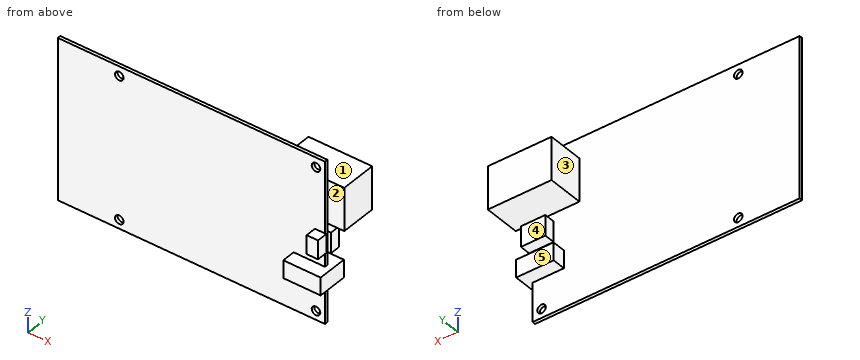
from build123d import *

# Parameters (mm, degrees)
ESQUISSE1_W             = 100
ESQUISSE1_H             = 60
BOSS_EXTRU_1_DEPTH      = 1.2
ESQUISSE2_W             = 21.84
ESQUISSE2_H             = 16
BOSS_EXTRU_2_DEPTH      = 13.5
ESQUISSE3_W             = 9.16
ESQUISSE3_H             = 7.62
BOSS_EXTRU_3_DEPTH      = 4
BOSS_EXTRU_4_DEPTH      = 5
BOSS_EXTRU_4_DEPTH_BACK = 6.2
ESQUISSE4_W             = 14
ESQUISSE4_H             = 6.6
ESQUISSE5_W             = 4.25
ESQUISSE5_H             = 7
BOSS_EXTRU_5_DEPTH      = 4
ENL_V_MAT_EXTRU_1_REACH = 119.398
ESQUISSE6_R             = 1.6
ESQUISSE7_W             = 16
ESQUISSE7_H             = 13.5
BOSS_EXTRU_6_DEPTH      = 2


with BuildPart() as part:
    # Esquisse1 → Boss.-Extru.1 (new body)
    with BuildSketch(Plane(origin=(0, 0, 0), x_dir=(1, 0, 0), z_dir=(0, 1, 0))):
        with Locations((-50, 30)):
            Rectangle(ESQUISSE1_W, ESQUISSE1_H)
    extrude(amount=-BOSS_EXTRU_1_DEPTH)

    # Esquisse2 → Boss.-Extru.2 (add)
    with BuildSketch(Plane(origin=(0, 0, 0), x_dir=(1, 0, 0), z_dir=(0, 1, 0))):
        with Locations((-6.62, 15.5)):
            Rectangle(ESQUISSE2_W, ESQUISSE2_H)
    extrude(amount=BOSS_EXTRU_2_DEPTH)

    # Esquisse3 → Boss.-Extru.3 (add)
    with BuildSketch(Plane(origin=(0, 0, 0), x_dir=(1, 0, 0), z_dir=(0, 1, 0))):
        with Locations((-3.29, 30.18)):
            Rectangle(ESQUISSE3_W, ESQUISSE3_H)
    extrude(amount=BOSS_EXTRU_3_DEPTH)

    # Esquisse4 → Boss.-Extru.4 (add, two sides: drawn at the far end of the back side and taken through both)
    with BuildSketch(Plane(origin=(0, 0, 0), x_dir=(1, 0, 0), z_dir=(0, 1, 0)).offset(-BOSS_EXTRU_4_DEPTH_BACK)):
        with Locations((-4.736, 42.16)):
            Rectangle(ESQUISSE4_W, ESQUISSE4_H)
    extrude(amount=BOSS_EXTRU_4_DEPTH + BOSS_EXTRU_4_DEPTH_BACK)

    # Esquisse5 → Boss.-Extru.5 (add)
    with BuildSketch(Plane.XZ.offset(1.2)):
        with Locations((-1.625, -30.01)):
            Rectangle(ESQUISSE5_W, ESQUISSE5_H)
    extrude(amount=BOSS_EXTRU_5_DEPTH)

    # Esquisse6 → Enlèv. mat.-Extru.1 (cut, up to next)
    with BuildSketch(Plane(origin=(0, 0, 0), x_dir=(1, 0, 0), z_dir=(0, 1, 0)), mode=Mode.PRIVATE) as enl_v_mat_extru_1_sk1:
        with Locations(Location((-77, 56.673, 0), (0, 0, 270))):
            Circle(ESQUISSE6_R)
    enl_v_mat_extru_1_tool1 = extrude(enl_v_mat_extru_1_sk1.sketch, amount=-ENL_V_MAT_EXTRU_1_REACH, mode=Mode.PRIVATE) & part.part
    # Esquisse6 → Enlèv. mat.-Extru.1 (cut, up to next)
    with BuildSketch(Plane(origin=(0, 0, 0), x_dir=(1, 0, 0), z_dir=(0, 1, 0)), mode=Mode.PRIVATE) as enl_v_mat_extru_1_sk2:
        with Locations(Location((-77, 3.581, 0), (0, 0, 270))):
            Circle(ESQUISSE6_R)
    enl_v_mat_extru_1_tool2 = extrude(enl_v_mat_extru_1_sk2.sketch, amount=-ENL_V_MAT_EXTRU_1_REACH, mode=Mode.PRIVATE) & part.part
    # Esquisse6 → Enlèv. mat.-Extru.1 (cut, up to next)
    with BuildSketch(Plane(origin=(0, 0, 0), x_dir=(1, 0, 0), z_dir=(0, 1, 0)), mode=Mode.PRIVATE) as enl_v_mat_extru_1_sk3:
        with Locations(Location((-3.35, 56.673, 0), (0, 0, 270))):
            Circle(ESQUISSE6_R)
    enl_v_mat_extru_1_tool3 = extrude(enl_v_mat_extru_1_sk3.sketch, amount=-ENL_V_MAT_EXTRU_1_REACH, mode=Mode.PRIVATE) & part.part
    # Esquisse6 → Enlèv. mat.-Extru.1 (cut, up to next)
    with BuildSketch(Plane(origin=(0, 0, 0), x_dir=(1, 0, 0), z_dir=(0, 1, 0)), mode=Mode.PRIVATE) as enl_v_mat_extru_1_sk4:
        with Locations(Location((-3.349, 3.581, 0), (0, 0, 270))):
            Circle(ESQUISSE6_R)
    enl_v_mat_extru_1_tool4 = extrude(enl_v_mat_extru_1_sk4.sketch, amount=-ENL_V_MAT_EXTRU_1_REACH, mode=Mode.PRIVATE) & part.part
    add(enl_v_mat_extru_1_tool1.solids().sort_by_distance((-77, 0, -56.673))[0], mode=Mode.SUBTRACT)
    add(enl_v_mat_extru_1_tool2.solids().sort_by_distance((-77, 0, -3.581))[0], mode=Mode.SUBTRACT)
    add(enl_v_mat_extru_1_tool3.solids().sort_by_distance((-3.35, 0, -56.673))[0], mode=Mode.SUBTRACT)
    add(enl_v_mat_extru_1_tool4.solids().sort_by_distance((-3.349, 0, -3.581))[0], mode=Mode.SUBTRACT)

    # Esquisse7 → Boss.-Extru.6 (add)
    with BuildSketch(Plane(origin=(4.3, 0, 0), x_dir=(0, 0, -1), z_dir=(1, 0, 0))):
        with Locations((15.5, 6.75)):
            Rectangle(ESQUISSE7_W, ESQUISSE7_H)
    extrude(amount=BOSS_EXTRU_6_DEPTH)


solid = part.part
For this review, take the finished solid that the model builds, in its own axes (mm). Face numbers are marked on the shaded views. A direction names the side the tool comes from. Coordinates: 2 decimals unless noted, no trailing zeros. Order: outer loops, then holes, each group sorted by start corner. A loop starts at its lowest first (then second) coordinate and runs counter-clockwise, first axis right, second up. Notation, with made-up numbers: (42.25, 25.5) - (87.25, 25.5) arc R37 cw to (87.25, 64.5) - close; hole circle Ø2 at (41, 3.25). An arc over 180 degrees is marked (long way). Answer as CSV lines item,"result". Start each with the question number.
1) Add section C-C (x = -10). State the section outline as (y, z) points, then the cut area to 3 significant figures.
2) Insertion check: P1, Ø12, axis at x = -54.5, z = -44.5, coming from the -Y side; P2, Ø4, axis at x = -6.5, y = 10, coming from the +Z side; P3, Ø4.5, axis at x = -1, z = -28.5, coming from the -Y side; P4, Ø4.5, axis at x = -2, y = -3, coming from the +Z side. Each pin has a flat end and moves straight along its axis. Give the tip position at first contact, or say it passes through.
3) To check wall thickness, follow line 1 along Z through (x, y) = (-77, -0.6); line 2 along Y through (x, z) = (-92, -23); line 3 along X through (y, z) = (3.75, -43). State the ranges of each line that lie inside material, in increasing order. Write a range as [from, to].
4) Add section D-D (y = 10). State the section outline as (x, z) points.
5) Add section B-B (y = -2.75). State the section outline as (x, z) points, then the cut area to 3 significant figures.
6) Add section A-A (x = -77). State the section outline as (y, z) points, then the cut area to 3 significant figures.
7) Machinability: for the marked faces 1, 2, 3, 4 and 5, which of the approach directions +Z, -Z, +X, -X, +Y, -Y give a long, thin tool a straight path to every point of the face, cutting with its end or side? Answer none if there is none.
Result:
1,outline,"(-6.2, -45.46) - (-1.2, -45.46) - (-1.2, -60) - (0, -60) - (0, -45.46) - (5, -45.46) - (5, -38.86) - (0, -38.86) - (0, -23.5) - (13.5, -23.5) - (13.5, -7.5) - (0, -7.5) - (0, 0) - (-1.2, 0) - (-1.2, -38.86) - (-6.2, -38.86) - close"
1,area,"354 mm^2"
2,P1,"y = -1.2"
2,P2,"z = -7.5"
2,P3,"y = -5.2"
2,P4,"z = 0"
3,line 1,"[-60, -58.27], [-55.07, -5.18], [-1.98, 0]"
3,line 2,"[-1.2, 0]"
3,line 3,"[-11.74, 2.26]"
4,outline,"(-17.54, -23.5) - (6.3, -23.5) - (6.3, -7.5) - (-17.54, -7.5) - close"
5,outline,"(-11.74, -45.46) - (2.26, -45.46) - (2.26, -38.86) - (-11.74, -38.86) - close; (-3.75, -33.51) - (0.5, -33.51) - (0.5, -26.51) - (-3.75, -26.51) - close"
5,area,"122 mm^2"
6,outline,"(-1.2, -60) - (0, -60) - (0, -58.27) - (-1.2, -58.27) - close; (-1.2, -55.07) - (0, -55.07) - (0, -5.18) - (-1.2, -5.18) - close; (-1.2, -1.98) - (0, -1.98) - (0, 0) - (-1.2, 0) - close"
6,area,"64.3 mm^2"
7,face 1,"+Z, +X, -X, +Y"
7,face 2,"+Z, +X, -Y"
7,face 3,"+Z, -Z, -X, +Y"
7,face 4,"+X, -X, +Y"
7,face 5,"-Z, +X, -X, +Y"
